Verification items for the finished model (mm, model axes). A direction names the side the tool comes from. Round coordinates to 2 decimals unless told otherwise and drop trailing zeros. Write each loop counter-clockwise with the first axis right and the second up, starting at its lowest first coordinate (ties: lowest second). Pieces come first, ordered by that corner, then holes. Notation, with made-up numbers: (-34, 77) -> (-11, 77) arc R20 ccw to (-11, 116) -> close; hole circle Ø1 at (23.5, 61.25). An arc over 180 degrees is marked (long way). Use CSV: the item, a comma, the result in double quotes.
```python
from build123d import *

# Parameters (mm, degrees)
SKETCH1_W           = 79.1
SKETCH1_H           = 30.7
BOSS_EXTRUDE1_DEPTH = 5.3
FILLET1_R           = 2
SKETCH2_W           = 4.3
SKETCH2_H           = 30.7
CUT_EXTRUDE1_DEPTH  = 4.8
BOSS_EXTRUDE2_DEPTH = 0.1


with BuildPart() as part:
    # Sketch1 → Boss-Extrude1 (new body)
    with BuildSketch(Plane(origin=(0, 0, 0), x_dir=(1, 0, 0), z_dir=(0, 1, 0))):
        Rectangle(SKETCH1_W, SKETCH1_H)
    extrude(amount=BOSS_EXTRUDE1_DEPTH)

    # Fillet1
    fillet1_edges = [part.edges().sort_by_distance(p)[0] for p in [
        (0, 5.3, -15.35),
        (0, 0, -15.35),
        (0, 0, 15.35),
        (0, 5.3, 15.35),
    ]]
    fillet(fillet1_edges, radius=FILLET1_R)

    # Sketch2 → Cut-Extrude1 (cut)
    with BuildSketch(Plane(origin=(0, 5.3, 0), x_dir=(1, 0, 0), z_dir=(0, 1, 0))):
        with Locations((37.4, 0)):
            Rectangle(SKETCH2_W, SKETCH2_H)
    extrude(amount=-CUT_EXTRUDE1_DEPTH, mode=Mode.SUBTRACT)

    # Sketch3 → Boss-Extrude2 (add, symmetric)
    with BuildSketch(Plane(origin=(0, 0.25, 0), x_dir=(1, 0, 0), z_dir=(0, 1, 0))):
        Polygon((39.55, 8.5), (41.55, 8.5), (41.55, 7.65), (43.65, 7.65), (43.65, 9), (47.05, 9), (47.05, 7.65), (48.05, 7.65), (48.05, 2.35), (47.05, 2.35), (47.05, 1), (43.65, 1), (43.65, 2.35), (41.55, 2.35), (41.55, 1.5), (39.55, 1.5), align=None)
    boss_extrude2 = extrude(amount=BOSS_EXTRUDE2_DEPTH, both=True)

    # Mirror1: Boss-Extrude2 across plane
    add(boss_extrude2.mirror(Plane.XY))


solid = part.part
```
Q1. Go/stop test with flat-tipped pins: P1, Ø1.3, axis at x = 38.5, z = 2, coming from the +Y side; P2, Ø2.5, axis at x = 44, z = 4.5, coming from the -Y side; P3, Ø9, axis at x = 45.5, z = -5.5, coming from the +Y side. Record where each tip stops, or that it passes through.
Filled in:
P1,"y = 0.5"
P2,"y = 0.15"
P3,"y = 0.35"
Q2. Material ranges on L1, parallel to X at y = 3.9, z = 6; L2, parallel to Z at x = 34, y = 1.8; L3, parallel to Z at x = -10, y = 4.05, recorded low to high.
Filled in:
L1,"-39.55 to 35.25"
L2,"-15.34 to 15.34"
L3,"-15.2 to 15.2"
Q3. Section check A-A (z = 6). Record the cut outline in (x, y).
Filled in:
outline,"(-39.55, 0) -> (39.55, 0) -> (39.55, 0.15) -> (48.05, 0.15) -> (48.05, 0.35) -> (39.55, 0.35) -> (39.55, 0.5) -> (35.25, 0.5) -> (35.25, 5.3) -> (-39.55, 5.3) -> close"
Q4. Section check B-B (x = 4). Record the cut outline in (y, z), plus the area to 3 significant figures.
Filled in:
outline,"(0, -13.35) arc R2 ccw to (2, -15.35) -> (3.3, -15.35) arc R2 ccw to (5.3, -13.35) -> (5.3, 13.35) arc R2 ccw to (3.3, 15.35) -> (2, 15.35) arc R2 ccw to (0, 13.35) -> close"
area,"159 mm²"
Q5. Access from +Z, -Z, +X, -X, +Y, -Y to the whole of each face (thin tool, end or side, straight path). Record for faces 1 (the flat face through (-39.55, 3, 0)), 2 (the flat face through (44, 0.15, -5)), 3 (the flat face through (35.25, 3, 0)).
Filled in:
face 1,"+Z, -Z, -X, +Y, -Y"
face 2,"+Z, -Z, +X, -Y"
face 3,"+Z, -Z, +X, +Y"
